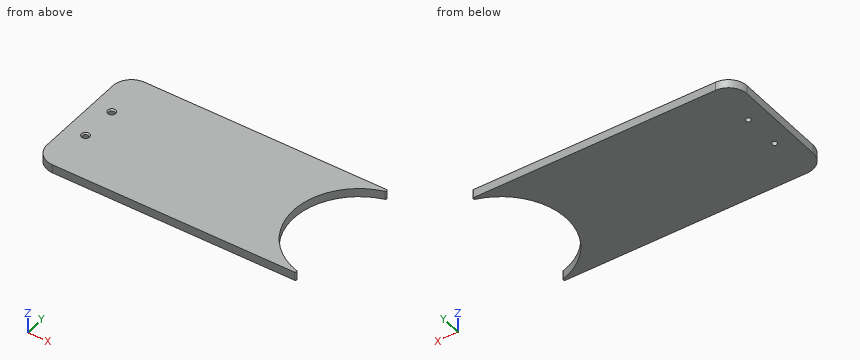
Autodesk Inventor part; units mm, degrees
ref_plane "YZ Plane" through (0, 0, 0) normal (1, 0, 0) x (0, 1, 0)
ref_plane "XZ Plane" through (0, 0, 0) normal (0, 1, 0) x (-1, 0, 0)
ref_plane "XY Plane" through (0, 0, 0) normal (0, 0, 1) x (1, 0, 0)
sketch "Эскиз1" plane through (0, 0, 0) normal (0, 0, 1) x (1, 0, 0)
  line L0 (52.25, 12.25) -> (0, 12.25)
  line L1 (0, -12.25) -> (52.25, -12.25)
  arc A0 (52.25, 12.25) -> (52.25, -12.25) centre (52.25, 0) ccw
  line L2 (0, -12.25) -> (0, 12.25)
  line L3 (0, 0) -> (40, 0) construction
  line L4 (0, 0) -> (0, 12.25) construction
  line L5 (0, 12.25) -> (0, 11.25)
  point P0 (20, 0)
  dimension "d0" = 12.25
  dimension "d47" = 40
extrude "Выдавливание3" add sketch "Эскиз1" along normal blind 1.6
fillet "Сопряжение3" radius 0.25 2 edges at (52.25, 12.25, 0.8) (52.25, -12.25, 0.8)
fillet "Сопряжение4" radius 3.5 2 edges at (0, -12.25, 0.8) (0, 12.25, 0.8)
sketch "Эскиз6" plane through (0, 0, 1.6) normal (0, 0, 1) x (1, 0, 0)
  arc A0 (48.82, 11.76) -> (48.82, -11.76) centre (52.25, 0) ccw construction
  line L0 (40, 0) -> (0, 0) construction
  line L1 (0, -12.25) -> (0, 12.25) construction
  circle A1 centre (3.5, 3.5) radius 0.5
  line L2 (3.5, 3.5) -> (0, 3.5) construction
  line L3 (3.5, 3.5) -> (3.5, 0) construction
  circle A2 centre (3.5, -3.5) radius 0.5
  point P0 (48.75, -12.25)
  dimension "d58" = 1
  dimension "d59" = 3.5
hole "Отверстие1" at (3.5, -3.5, 1.6) at (3.5, 3.5, 1.6) direction (0, 0, -1) diameter 1 end through all countersink diameter 1.5 countersink angle 90
properties part number "Поршень"
Can you work these out from the model? Positions are in its coordinate system, mm. Give positions to 0.01 mm unless a question says otherwise; leave off trailing zeros. Order: outer loops, then holes, each group sorted by start corner. A loop starts at its lowest first (then second) coordinate and runs counter-clockwise, first axis right, second up. Notation, with made-up numbers: M -32.75,81.25 L 9.25,81.25 A18 cw 9.25,97.25 Z; hole C 76.5,59.25 d1. An arc over 180 degrees is marked long. Use one line per item in the form item = value.
Item 1: If we section it at B-B, the plane y = 3.5: Write out the boundary of the cut face in (x, z), and give its area (3 significant figures).
Values follow:
outline = M 0,0 L 3,0 L 3,1.35 L 2.75,1.6 L 0,1.6 Z; M 4,0 L 40.51,0 L 40.51,1.6 L 4.25,1.6 L 4,1.35 Z
area = 63.2 mm^2
Item 2: If we section it at A-A, the plane z = 0.3: Write out the boundary of the cut face in (x, y).
Values follow:
outline = M 0,-8.75 A3.5 ccw 3.5,-12.25 L 48.75,-12.25 A0.25 ccw 48.82,-11.76 A12.25 cw 48.82,11.76 A0.25 ccw 48.75,12.25 L 3.5,12.25 A3.5 ccw 0,8.75 Z; hole C 3.5,-3.5 d1; hole C 3.5,3.5 d1
Item 3: If we section it at C-C, the plane x = 44: Write out the boundary of the cut face in (y, z).
Values follow:
outline = M -12.25,0 L -9.06,0 L -9.06,1.6 L -12.25,1.6 Z; M 9.06,0 L 12.25,0 L 12.25,1.6 L 9.06,1.6 Z
Item 4: If we section it at D-D, the plane y = 0: Write out the boundary of the cut face in (x, z).
Values follow:
outline = M 0,0 L 40,0 L 40,1.6 L 0,1.6 Z
Item 5: If I drill on line 1 along Y through (x, z) = (3.5, 0.2); line 2 along X through (y, z) = (3.5, 0.55); line 3 along Y through (x, z) = (44, 0.7), over which ranges is the centre line in solid material (lowest first)? Write a range as [from, to].
Values follow:
line_1 = [-12.25, -4], [-3, 3], [4, 12.25]
line_2 = [0, 3], [4, 40.51]
line_3 = [-12.25, -9.06], [9.06, 12.25]
